Autodesk Inventor part; units mm, degrees
ref_plane "YZ Plane" through (0, 0, 0) normal (1, 0, 0) x (0, 1, 0)
ref_plane "XZ Plane" through (0, 0, 0) normal (0, 1, 0) x (-1, 0, 0)
ref_plane "XY Plane" through (0, 0, 0) normal (0, 0, 1) x (1, 0, 0)
sketch "Náčrt1" plane through (0, 0, 0) normal (0, 0, 1) x (1, 0, 0)
  circle A0 centre (0, 0) radius 4
  arc A1 (0, 7) -> (0, -7) centre (0, 0) ccw
  line L0 (0, -9.8) -> (0, 9.8) construction
  line L1 (-14, 0) -> (35, 0) construction
  line L2 (0, -7) -> (28, -7)
  line L3 (28, -7) -> (28, -3)
  line L4 (28, -3) -> (20, -3)
  line L5 (20, -3) -> (20, 3)
  line L6 (20, 3) -> (28, 3)
  line L7 (28, 3) -> (28, 7)
  line L8 (28, 7) -> (0, 7)
  dimension "d0" = 8
  dimension "d1" = 14
  dimension "d2" = 4
  dimension "d3" = 4
  dimension "d4" = 6
  dimension "d5" = 8
  dimension "d6" = 28
extrude "Vysunutí1" add sketch "Náčrt1" along normal blind 8
sketch "Náčrt2" plane through (0, 0, 8) normal (0, 0, 1) x (1, 0, 0)
  line L0 (-14, 0) -> (35, 0) construction
  line L1 (0, -9.8) -> (0, 9.8) construction
  line L2 (8, 7) -> (16, 7)
  line L3 (16, 7) -> (16, -7)
  line L4 (16, -7) -> (8, -7)
  line L5 (8, -7) -> (8, 7)
  point P0 (0, 0)
  dimension "d10" = 8
  dimension "d11" = 8
  dimension "d12" = 7
  dimension "d13" = 7
extrude "Vysunutí2" add sketch "Náčrt2" along normal blind 5
sketch "Náčrt5" plane through (0, 0, 8) normal (0, 0, 1) x (1, 0, 0)
  line L0 (16, 7) -> (16, -7)
  line L1 (16, -7) -> (28, -7)
  line L2 (28, -7) -> (28, -3)
  line L3 (28, -3) -> (20, -3)
  line L4 (20, -3) -> (20, 3)
  line L5 (20, 3) -> (28, 3)
  line L6 (28, 3) -> (28, 7)
  line L7 (28, 7) -> (16, 7)
  point P0 (0, 0)
extrude "Vysunutí4" add sketch "Náčrt5" along normal blind 1
sketch "Náčrt6" plane through (0, -7, 0) normal (0, -1, 0) x (1, 0, 0)
  point P0 (0, 0)
fillet "Zaoblení2" radius 4.5 4 edges at (28, -5, 9) (28, -5, 0) (28, 5, 0) (28, 5, 9)
sketch "Náčrt7" plane through (0, -7, 0) normal (0, -1, 0) x (1, 0, 0)
  arc A0 (23.5, 0) -> (23.5, 9) centre (23.5, 4.5) ccw construction
  circle A1 centre (23.5, 4.5) radius 2
  point P0 (0, 0)
  dimension "d22" = 4
extrude "Vysunutí5" cut sketch "Náčrt7" against normal through all
properties part number "Součást15"
Work out the finished part from the listing and answer in its coordinate system (mm). A direction names the side the tool comes from. Coordinates: 2 decimals unless noted, no trailing zeros. Order: outer loops, then holes, each group sorted by start corner. A loop starts at its lowest first (then second) coordinate and runs counter-clockwise, first axis right, second up. Notation, with made-up numbers: (-29.75, 86.25) - (-24.75, 86.25) arc R18 cw to (-24.75, 106.25) - close; hole circle Ø11 at (-36, 45). An arc over 180 degrees is marked (long way). Put each result on its own line as item: value. Start each with the question number.
1) For a pull along Y with two mould halves and no side action, classify faces 5 (the flat face through (14, -7, 5)), 6 (the flat face through (12, 0, 13)), 7 (the flat face through (24, -3, 2)) as released by +Y, released by -Y, zero draft, split by the parting line, or undercut.
2) Find the intervals of material crossed by line 1 (Y direction, x = 22, z = 8.5); line 2 (Z direction, x = 18, y = -2.25); line 3 (X direction, y = -2.75, z = 5.75), in increasing order. Write a range as from..to.
3) Find section A-A (z = 5). Give the vertices of the cut face in (x, y).
4) Flat-ended cylindrical pins translate along their axes: pin 1 (3 mm diameter, centred on x = 2.5, y = 2.5, fed in from -Z); pin 2 (3 mm diameter, centred on y = -2, z = 8.5, fed in from -X); pin 3 (6 mm diameter, centred on x = 19.5, y = 3, fed in from +Z); pin 4 (2 mm diameter, centred on y = -2.5, z = 11.5, fed in from +X). Find the tip coordinate at first contact, or state that the pin passes through.
5) For faces 1 (the flat face through (16, 0, 11)), 2 (the flat face through (20, 0, 4)), 3 (the cylindrical face through (-7, 0, 4)), 4 (the flat face through (8, 0, 10)), determine the directions among +Z, -Z, +X, -X, +Y, -Y from which every point of the face is accessible in a straight line to the end or side of a thin tool.
6) Find section D-D (z = 1). Give the vertices of the cut face in (x, y), plus the area to 3 significant figures.
7) Find section B-B (x = 20.5). Give the vertices of the cut face in (y, z), plus the area to 3 significant figures.
Results list:
1. face 5: released by -Y
1. face 6: zero draft
1. face 7: undercut
2. line 1: y = -7..-3, 3..7
2. line 2: z = 0..9
2. line 3: x = -6.44..-2.9, 2.9..20
3. outline: (0, -7) - (21.56, -7) - (21.56, -3) - (20, -3) - (20, 3) - (21.56, 3) - (21.56, 7) - (0, 7) arc R7 ccw to start; (25.44, -7) - (27.97, -7) - (27.97, -3) - (25.44, -3) - close; (25.44, 3) - (27.97, 3) - (27.97, 7) - (25.44, 7) - close; hole circle Ø8 at (0, 0)
4. pin 1: stops at z = 0
4. pin 2: stops at x = -6.98
4. pin 3: stops at z = 9
4. pin 4: stops at x = 16
5. face 1: +Z, +X, +Y, -Y
5. face 2: +Z, -Z, +X
5. face 3: +Z, -Z, -X
5. face 4: +Z, -X, +Y, -Y
6. outline: (0, -7) - (26.33, -7) - (26.33, -3) - (20, -3) - (20, 3) - (26.33, 3) - (26.33, 7) - (0, 7) arc R7 ccw to start; hole circle Ø8 at (0, 0)
6. area: 357 mm^2
7. outline: (-7, 0) - (-3, 0) - (-3, 9) - (-7, 9) - close; (3, 0) - (7, 0) - (7, 9) - (3, 9) - close
7. area: 72.0 mm^2
